```python
from build123d import *

# Parameters (mm, degrees)
SKETCH1_R                                 = 6
BOSS_EXTRUDE1_DEPTH                       = 4
SKETCH2_R                                 = 4
BOSS_EXTRUDE2_DEPTH                       = 6
F_2_0MM_PRESS_DOWEL_HOLE1_D               = 2
F_2_0MM_PRESS_DOWEL_HOLE1_DEPTH           = 3.25
F_2_0MM_PRESS_DOWEL_HOLE1_TIP             = 0.600860619
F_2_0MM_PRESS_DOWEL_HOLE1_ON_FACE_2_D     = 2
F_2_0MM_PRESS_DOWEL_HOLE1_ON_FACE_2_DEPTH = 3.25
F_2_0MM_PRESS_DOWEL_HOLE1_ON_FACE_2_TIP   = 0.600860619
CUT_EXTRUDE1_DEPTH                        = 14.114877125
CUT_EXTRUDE1_DEPTH_BACK                   = 14.114877125
SKETCH8_W                                 = 1.5
SKETCH8_H                                 = 6


with BuildPart() as part:
    # Sketch1 → Boss-Extrude1 (new, symmetric)
    with BuildSketch(Plane(origin=(0, 0, 0), x_dir=(1, 0, 0), z_dir=(0, 1, 0))):
        with Locations(Location((0, 0, 0), (0, 0, 270))):
            Circle(SKETCH1_R)
    extrude(amount=BOSS_EXTRUDE1_DEPTH, both=True)

    # Sketch2 → Boss-Extrude2 (add)
    with BuildSketch(Plane.XZ.offset(4)):
        with Locations(Location((0, 0, 0), (0, 0, 270))):
            Circle(SKETCH2_R)
    extrude(amount=BOSS_EXTRUDE2_DEPTH)

    # Ø2.0mm Press Dowel Hole1
    with Locations(Plane(origin=(0, -7.5, 4), x_dir=(1, 0, 0), z_dir=(0, 0, 1))):
        with Locations((0, 0)):
            Hole(F_2_0MM_PRESS_DOWEL_HOLE1_D / 2, depth=F_2_0MM_PRESS_DOWEL_HOLE1_DEPTH)
            with Locations((0, 0, -(F_2_0MM_PRESS_DOWEL_HOLE1_DEPTH + F_2_0MM_PRESS_DOWEL_HOLE1_TIP / 2))):  # 118° drill point
                Cone(0, F_2_0MM_PRESS_DOWEL_HOLE1_D / 2, F_2_0MM_PRESS_DOWEL_HOLE1_TIP, mode=Mode.SUBTRACT)

    # Ø2.0mm Press Dowel Hole1 on face 2
    with Locations(Plane(origin=(0, -7.5, -4), x_dir=(-1, 0, 0), z_dir=(0, 0, -1))):
        with Locations((0, 0)):
            Hole(F_2_0MM_PRESS_DOWEL_HOLE1_ON_FACE_2_D / 2, depth=F_2_0MM_PRESS_DOWEL_HOLE1_ON_FACE_2_DEPTH)
            with Locations((0, 0, -(F_2_0MM_PRESS_DOWEL_HOLE1_ON_FACE_2_DEPTH + F_2_0MM_PRESS_DOWEL_HOLE1_ON_FACE_2_TIP / 2))):  # 118° drill point
                Cone(0, F_2_0MM_PRESS_DOWEL_HOLE1_ON_FACE_2_D / 2, F_2_0MM_PRESS_DOWEL_HOLE1_ON_FACE_2_TIP, mode=Mode.SUBTRACT)

    # Sketch8 → Cut-Extrude1 (cut, two sides: drawn at the far end of the back side and taken through both)
    with BuildSketch(Plane(origin=(0, 0, 0), x_dir=(0, 0, -1), z_dir=(1, 0, 0)).offset(-CUT_EXTRUDE1_DEPTH_BACK)):
        with Locations((0, -7)):
            Rectangle(SKETCH8_W, SKETCH8_H)
    extrude(amount=CUT_EXTRUDE1_DEPTH + CUT_EXTRUDE1_DEPTH_BACK, mode=Mode.SUBTRACT)


solid = part.part
```
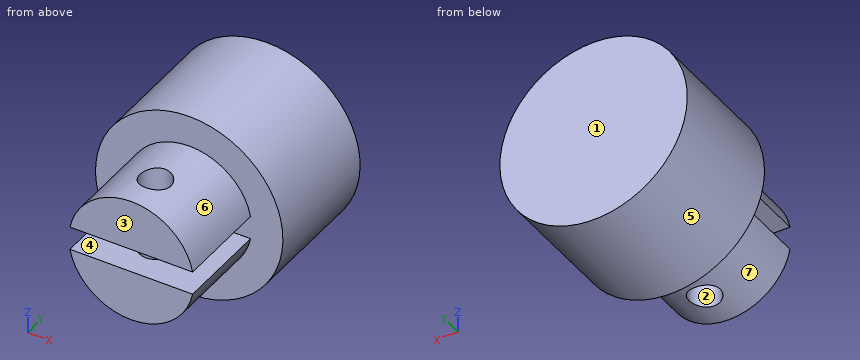
Here's how the part is built. I have some questions about the finished solid (model axes, mm). Face numbers are marked on the shaded views. A direction names the side the tool comes from. Coordinates: 2 decimals unless noted, no trailing zeros. Order: outer loops, then holes, each group sorted by start corner. A loop starts at its lowest first (then second) coordinate and runs counter-clockwise, first axis right, second up.
1) Which directions (+Z, -Z, +X, -X, +Y, -Y) give clear straight access to the entire face, cutting with the end or side of a thin tool? Please do the marked faces 5, 6 and 7.
2) We'd pull the mould along Y, two halves only. Please class the marked faces 1, 2, 3 and 4: +Y half, -Y half, draft (parallel to the pull), parting line (faces both ways), or undercut.
3) Will these pins go through, and if not, where does the flat tip stop? pin 1 (2.5 mm diameter, centred on x = 0, y = -7.5, fed in from +Z); pin 2 (5 mm diameter, centred on x = -3, y = -8.5, fed in from -Z); pin 3 (1.5 mm diameter, centred on y = 2, z = -4.5, fed in from -X); pin 4 (1.8 mm diameter, centred on x = 0, y = -7.5, fed in from -Z).
4) Imagine slicing it at A-A on x = 0. List the corners of the cut face in (y, z) for me, and give its area (3 significant figures).
5) Imagine slicing it at B-B on y = -7.5. List the corners of the cut face in (x, z) for me.
6) Imagine slicing it at C-C on z = -1. List the corners of the cut face in (x, y) for me, and give its area (3 significant figures).
7) Imagine slicing it at D-D on y = -2.75. List the corners of the cut face in (x, z) for me.
8) I need wall thicknesses on line 1 (Y direction, x = 0, z = -3.2); line 2 (Y direction, x = -3.25, z = -3.5); line 3 (Z direction, x = 2, y = -4.5). Which ranges of each line are inside material? Lowest first, please.
Response values:
1. face 5: +Y, -Y
1. face 6: +Z, -Y
1. face 7: -Z, -Y
2. face 1: +Y half
2. face 2: undercut
2. face 3: -Y half
2. face 4: draft
3. pin 1: stops at z = 4
3. pin 2: stops at z = -3.97
3. pin 3: stops at x = -4.68
3. pin 4: passes through
4. outline: (-10, -4) - (-8.5, -4) - (-8.5, -0.75) - (-10, -0.75) - close; (-10, 0.75) - (-8.5, 0.75) - (-8.5, 4) - (-10, 4) - close; (-6.5, -4) - (-4, -4) - (-4, -6) - (4, -6) - (4, 6) - (-4, 6) - (-4, 4) - (-6.5, 4) - (-6.5, 0.75) - (-4, 0.75) - (-4, -0.75) - (-6.5, -0.75) - close
4. area: 122 mm2
5. outline: (-3.93, -0.75) arc R4 ccw to (-1, -3.87) - (-1, -0.75) - close; (-3.93, 0.75) - (-1, 0.75) - (-1, 3.87) arc R4 ccw to start; (1, -3.87) arc R4 ccw to (3.93, -0.75) - (1, -0.75) - close; (1, 0.75) - (3.93, 0.75) arc R4 ccw to (1, 3.87) - close
6. outline: (-5.92, -4) - (-3.87, -4) - (-3.87, -10) - (3.87, -10) - (3.87, -4) - (5.92, -4) - (5.92, 4) - (-5.92, 4) - close; hole circle Ø2 at (0, -7.5)
6. area: 138 mm2
7. outline: circle Ø12 at (0, 0)
8. line 1: y = -10 to -8.5, -6.5 to 4
8. line 2: y = -4 to 4
8. line 3: z = -3.46 to -0.75, 0.75 to 3.46
